```python
from build123d import *

# Parameters (mm, degrees)
F0_W     = 58.472368
F0_H     = 64.15464
F1_DEPTH = 44.45
F2_W     = 50.716958
F2_H     = 26.597259
F2_H_2   = 21.220153
F3_DEPTH = 42.926
F4_W     = 4.469927
F4_H     = 4.469931
F4_W_2   = 4.624061
F4_H_2   = 4.46993
F4_W_3   = 4.007522
F4_W_4   = 4.31579
F4_H_3   = 4.315794
F5_DEPTH = 1.524
F6_R     = 6.469246
F7_DEPTH = 2.4384
F8_W     = 1.37474
F8_H     = 3.070258
F8_W_2   = 1.374744
F8_H_2   = 2.978608
F8_W_3   = 1.328919
F9_DEPTH = 2.794


with BuildPart() as f1:
    # F0 (on Front) → F1 (new body)
    with BuildSketch(Plane.XZ):
        Rectangle(F0_W, F0_H)
    extrude(amount=F1_DEPTH)

    # F2 (on face) → F3 (cut)
    with BuildSketch(Plane.XZ.offset(44.45)):
        with Locations((0, -14.125422)):
            Rectangle(F2_W, F2_H)
        with Locations((0, 16.780822)):
            Rectangle(F2_W, F2_H_2)
    extrude(amount=-F3_DEPTH, mode=Mode.SUBTRACT)

    # F4 (on face) → F5 (join)
    with BuildSketch(Plane(origin=(0, 0, -32.07732), x_dir=(1, 0, 0), z_dir=(0, 0, -1))):
        with Locations((-25.636799, 41.048552)):
            Rectangle(F4_W, F4_H)
        with Locations((-25.636799, 3.747775)):
            Rectangle(F4_W_2, F4_H_2)
        with Locations((24.996694, 3.747775)):
            Rectangle(F4_W_3, F4_H_2)
        with Locations((24.996694, 41.048553)):
            Rectangle(F4_W_4, F4_H_3)
    extrude(amount=F5_DEPTH)

    # F6 (on face) → F7 (cut)
    with BuildSketch(Plane.XY.offset(32.07732)):
        with Locations((19.203754, -36.686223)):
            Circle(F6_R)
    extrude(amount=-F7_DEPTH, mode=Mode.SUBTRACT)

    # F8 (on face) → F9 (cut)
    with BuildSketch(Plane.YZ.offset(29.236184)):
        with Locations((-37.546458, 29.409513)):
            Rectangle(F8_W, F8_H)
        with Locations((-40.158469, 29.455338)):
            Rectangle(F8_W_2, F8_H_2)
        with Locations((-42.655916, 29.455338)):
            Rectangle(F8_W_3, F8_H_2)
    extrude(amount=-F9_DEPTH, mode=Mode.SUBTRACT)


solid = f1.part
```
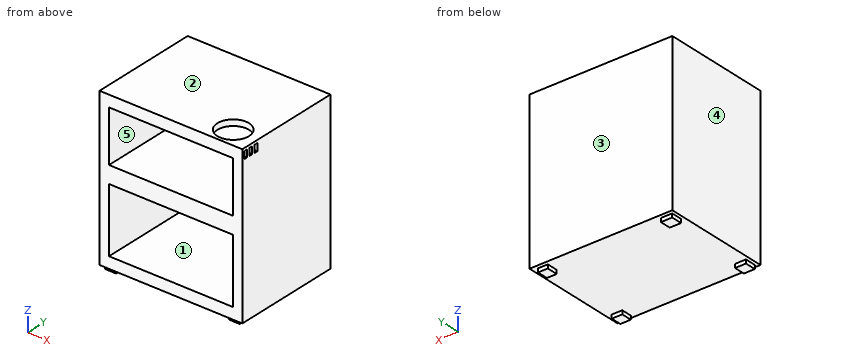
Work out the finished part from the listing and answer in its coordinate system (mm). Face numbers are marked on the shaded views. A direction names the side the tool comes from. Give positions to 0.01 mm unless a question says otherwise; leave off trailing zeros. Write each loop counter-clockwise with the first axis right and the second up, starting at its lowest first coordinate (ties: lowest second). Pieces come first, ordered by that corner, then holes.
(1) The part is cut by section D-D on y = -32. Write down the section's boundary in (x, z), plus the area to 3 significant figures.
Final values:
outline: (-29.24, -32.08) - (29.24, -32.08) - (29.24, 32.08) - (23.66, 32.08) - (23.66, 29.64) - (14.74, 29.64) - (14.74, 32.08) - (-29.24, 32.08) - close; hole (-25.36, -27.42) - (25.36, -27.42) - (25.36, -0.83) - (-25.36, -0.83) - close; hole (-25.36, 6.17) - (25.36, 6.17) - (25.36, 27.39) - (-25.36, 27.39) - close
area: 1,300 mm2
(2) The part is cut by section C-C on z = 18.5. Write down the section's boundary in (x, y), plus the area to 3 significant figures.
Final values:
outline: (-29.24, -44.45) - (-25.36, -44.45) - (-25.36, -1.52) - (25.36, -1.52) - (25.36, -44.45) - (29.24, -44.45) - (29.24, 0) - (-29.24, 0) - close
area: 422 mm2
(3) Straight lines are drawn through the part: line 1 (Z direction, x = 0.5, y = -41); line 2 (X direction, y = -16.5, z = -26); line 3 (Z direction, x = 27, y = -18). For each, find the intervals that lie inside material, in ascending order.
Final values:
line 1: z = -32.08 to -27.42, -0.83 to 6.17, 27.39 to 32.08
line 2: x = -29.24 to -25.36, 25.36 to 29.24
line 3: z = -32.08 to 32.08
(4) Which of the six approach directions +Z, -Z, +X, -X, +Y, -Y give full straight-line access (tool end or side, diameter ignored) to the marked faces 4 and 5?
Final values:
face 4: +Z, -Z, -X, +Y, -Y
face 5: -Y
(5) The mould has two halves that part along Z. Classify the marked faces 1, 2 and 3: pulls with the +Z half, pulls with the -Z half, needs draft (parallel to the pull), parting line crosses it, or undercut.
Final values:
face 1: undercut
face 2: pulls with the +Z half
face 3: needs draft
(6) The part is cut by section A-A on y = -17.5. Write down the section's boundary in (x, z), plus the area to 3 significant figures.
Final values:
outline: (-29.24, -32.08) - (29.24, -32.08) - (29.24, 32.08) - (-29.24, 32.08) - close; hole (-25.36, -27.42) - (25.36, -27.42) - (25.36, -0.83) - (-25.36, -0.83) - close; hole (-25.36, 6.17) - (25.36, 6.17) - (25.36, 27.39) - (-25.36, 27.39) - close
area: 1,330 mm2
(7) The part is cut by section B-B on x = -9. Write down the section's boundary in (y, z), plus the area to 3 significant figures.
Final values:
outline: (-44.45, -32.08) - (0, -32.08) - (0, 32.08) - (-44.45, 32.08) - (-44.45, 27.39) - (-1.52, 27.39) - (-1.52, 6.17) - (-44.45, 6.17) - (-44.45, -0.83) - (-1.52, -0.83) - (-1.52, -27.42) - (-44.45, -27.42) - close
area: 799 mm2
(8) Flat-ended cylindrical pins translate along their axes: pin 1 Ø4 at (x, z) = (8, -3) entering from -Y; pin 2 Ø1.7 at (y, z) = (-40.5, -33) entering from +X; pin 3 Ø0.8 at (x, z) = (-24.5, -33) entering from -Y. Find the tip coordinate at first contact, or state that the pin passes through.
Final values:
pin 1: stops at y = -1.52
pin 2: stops at x = 27.15
pin 3: stops at y = -43.28
